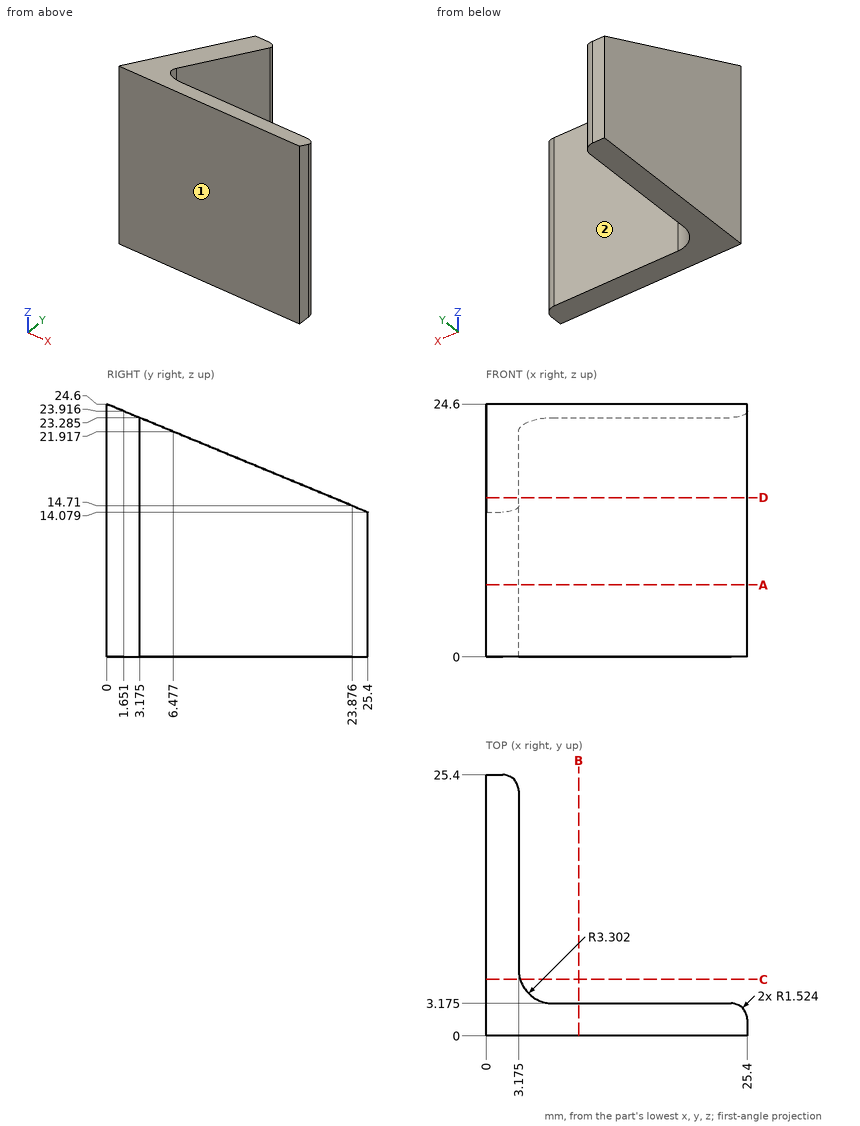
Verification items for this drawing (mm, ordinates from the low corner). A direction names the side the tool comes from. Coordinates: 2 decimals unless noted, no trailing zeros. Order: outer loops, then holes, each group sorted by start corner. A loop starts at its lowest first (then second) coordinate and runs counter-clockwise, first axis right, second up. Notation, with made-up numbers: M 19.5,59.5 L 59.5,59.5 A16 ccw 59.5,76.5 Z; hole C -21.5,20.5 d8. An arc over 180 degrees is marked long. One line per item, written item: value. Start each with the question number.
Item 1: Sectioned sample at A-A on z = 7. Record the cut outline in (x, y) (3 decimals).
Item 2: Depth check by flat-ended pin: P1, Ø12, axis at y = 18.5, z = 7, coming from the +X side (3 decimals); P2, Ø10, axis at x = 11.5, z = 2.5, coming from the +Y side (3 decimals); P3, Ø10, axis at y = 9, z = 11, coming from the -X side. Enter the tip coordinate at first touch or a pass-through.
Item 3: Access from +Z, -Z, +X, -X, +Y, -Y to the whole of each face (thin tool, end or side, straight path). Record for the marked faces 1 and 2.
Item 4: Sectioned sample at C-C on y = 5.5. Record the cut outline in (x, z).
Item 5: Sectioned sample at B-B on x = 9. Record the cut outline in (y, z) (1 decimal).
Item 6: Sectioned sample at D-D on z = 15.5. Record the cut outline in (x, y) (1 decimal).
Item 7: Thickness scan on probe 1 along X at (y, z) = (20, 15.5) (3 decimals); probe 2 along Y at (x, z) = (2.75, 7). Record the ranges inside material, lowest first.
Calculated:
1. outline: M 0,0 L 25.4,0 L 25.4,1.651 A1.524 ccw 23.876,3.175 L 6.477,3.175 A3.302 cw 3.175,6.477 L 3.175,23.876 A1.524 ccw 1.651,25.4 L 0,25.4 Z
2. P1: x = 3.175
2. P2: y = 3.175
2. P3: x = 0
3. face 1: +Z, -Z, +X, -X, -Y
3. face 2: +Z, -Z, +X, +Y
4. outline: M 0,0 L 3.32,0 L 3.32,22.32 L 0,22.32 Z
5. outline: M 0,0 L 3.2,0 L 3.2,23.3 L 0,24.6 Z
6. outline: M 0,0 L 25.4,0 L 25.4,1.7 A1.5 ccw 23.9,3.2 L 6.5,3.2 A3.3 cw 3.2,6.5 L 3.2,22 L 0,22 Z
7. probe 1: 0 to 3.175
7. probe 2: 0 to 24.93
